For this review, use the dimensioned drawing (mm, ordinates from the lowest corner) and the shaded views. A direction names the side the tool comes from. Give positions to 0.01 mm unless a question says otherwise; leave off trailing zeros. Write each question's results on one line, items separated by ' | '. Start each with the question number.
Q1. We need section A-A (y = 8.75). Give the number of separate pieces and of enclosed holes in the cut face.
Q2. Wall thickness on L1, parallel to Y at x = 8, z = 2.5 (1 decimal); L2, parallel to Y at x = 9.75, z = 4.25 (1 decimal); L3, parallel to X at y = 5.25, z = 2 (1 decimal): over which ranges is each line inside the solid? List them lowest first. Write a range as [from, to].
Q3. Insertion check: pin 1 Ø3 at (x, z) = (4.5, 1) entering from +Y; pin 2 Ø1 at (x, z) = (1.5, 2) entering from -Y; pin 3 Ø3.5 at (x, z) = (2, 1.5) entering from +Y. Each pin has a flat end and moves straight along its axis. Give the tip position at first contact, or say it passes through.
Q4. Mouldability with a two-part tool opening along X and no side actions: class the marked faces 3 and 4 as released by +X, released by -X, zero draft, split by the parting line, or undercut.
Q5. Machinability: for the marked faces 1 and 2, which of the approach directions +Z, -Z, +X, -X, +Y, -Y give a long, thin tool a straight path to every point of the face, cutting with its end or side? Answer none if there is none.
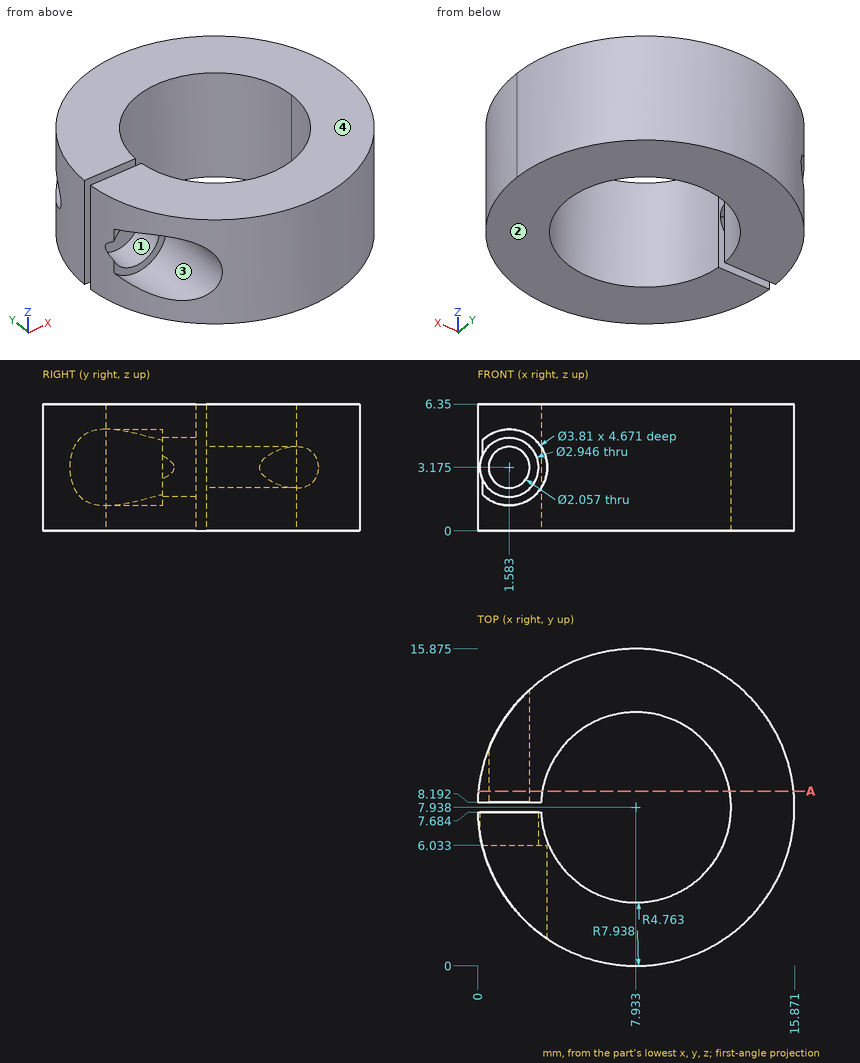
Output:
1) separate pieces: 2 | enclosed holes: 1
2) L1: [0, 3.2], [12.7, 15.9] | L2: [0.2, 3.5], [12.3, 15.7] | L3: [3.1, 4], [11.9, 15.4]
3) pin 1: y = 15.64 | pin 2: y = 6.03 | pin 3: y = 14.68
4) face 3: undercut | face 4: zero draft
5) face 1: -Y | face 2: -Z, +X, -X, +Y, -Y
